Input: dimensioned drawing with shaded views. Units: mm. Origin: part minimum x, y, z. A direction names the side the tool comes from. Give positions to 0.01 mm unless a question says otherwise; leave off trailing zeros. Loops run counter-clockwise (first coordinate to the right, second up) from the corner with the lowest first, then second, coordinate; pieces in that order, holes last.
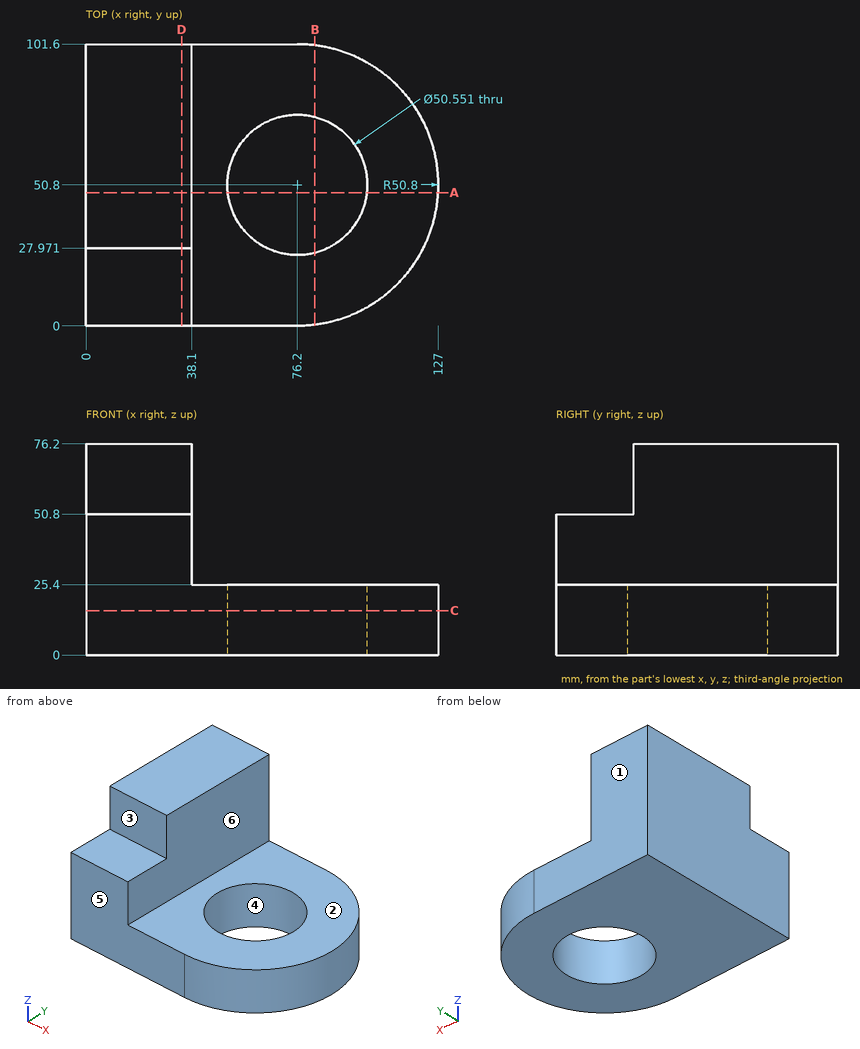
(1) Ray query, line 1 along Y through (x, z) = (76, 16) (1 decimal); line 2 along X through (y, z) = (50.8, 8.75); line 3 along X through (y, z) = (77.5, 42.5). Return the intervals inside material, ascending.
A:
line 1: y = 0 to 25.5, 76.1 to 101.6
line 2: x = 0 to 50.92, 101.48 to 127
line 3: x = 0 to 38.1
(2) Section B-B, the plane x = 82.5. Return the cut outline in (y, z).
A:
outline: (0.39, 0) - (26.32, 0) - (26.32, 25.4) - (0.39, 25.4) - close; (75.28, 0) - (101.21, 0) - (101.21, 25.4) - (75.28, 25.4) - close
(3) Section A-A, the plane y = 48. Return the cut outline in (x, z).
A:
outline: (0, 0) - (51.08, 0) - (51.08, 25.4) - (38.1, 25.4) - (38.1, 76.2) - (0, 76.2) - close; (101.32, 0) - (126.92, 0) - (126.92, 25.4) - (101.32, 25.4) - close
(4) Reachability of the marked faces 1, 2 and 3 from +Z, -Z, +X, -X, +Y, -Y: full face, straight path, thin tool, end or side. Return the list, or none.
A:
face 1: +Z, -Z, +X, -X, +Y
face 2: +Z, +X, +Y, -Y
face 3: +Z, +X, -X, -Y
(5) Mould query, pull axis Y, two halves, no side actions, for the marked faces 4, 5 and 6. Classes: pulls with the +Y half, pulls with the -Y half, needs draft (parallel to the pull), parting line crosses it, or undercut.
A:
face 4: undercut
face 5: pulls with the -Y half
face 6: needs draft
(6) First-contact query: pin 1 (3 mm diameter, centred on y = 89.5, z = 48, fed in from -X); pin 2 (5 mm diameter, centred on y = 49.5, z = 45, fed in from +X); pin 3 (20.5 mm diameter, centred on x = 14, z = 64, fed in from -Y); pin 4 (10 mm diameter, centred on y = 18, z = 22.5, fed in from +X). Flat tips, straight axial feed; report the tip coordinate or a pass-through.
A:
pin 1: stops at x = 0
pin 2: stops at x = 38.1
pin 3: stops at y = 27.97
pin 4: stops at x = 118.72
(7) Section D-D, the plane x = 34.5. Return the cut outline in (y, z).
A:
outline: (0, 0) - (101.6, 0) - (101.6, 76.2) - (27.97, 76.2) - (27.97, 50.8) - (0, 50.8) - close
(8) Section C-C, the plane z = 16. Return the cut outline in (x, y).
A:
outline: (0, 0) - (76.2, 0) arc R50.8 ccw to (76.2, 101.6) - (0, 101.6) - close; hole circle Ø50.55 at (76.2, 50.8)
